Verification items for the finished model (mm, model axes). Give positions to 0.01 mm unless a question says otherwise; leave off trailing zeros. Write each loop counter-clockwise with the first axis right and the second up, starting at its lowest first coordinate (ties: lowest second). Pieces come first, ordered by that corner, then holes. Notation, with made-up numbers: (51.5, 63.5) -> (94.5, 63.5) arc R28 ccw to (94.5, 84.5) -> close; hole circle Ø7 at (71.5, 68.25). An arc over 180 degrees is marked (long way). Write item = value, one per line.
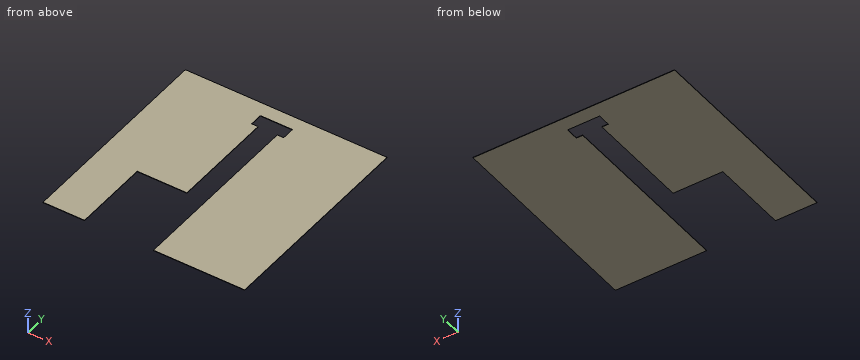
from build123d import *

# Parameters (mm, degrees)
CROQUIS1_W              = 1258.4
CROQUIS1_H              = 1300
SALIENTE_EXTRUIR1_DEPTH = 2.9
CROQUIS2_W              = 200
CROQUIS2_H              = 80
CORTAR_EXTRUIR1_DEPTH   = 10
CORTAR_EXTRUIR2_DEPTH   = 3


with BuildPart() as part:
    # Croquis1 → Saliente-Extruir1 (new body)
    with BuildSketch(Plane.XY):
        with Locations((629.2, -650)):
            Rectangle(CROQUIS1_W, CROQUIS1_H)
    extrude(amount=SALIENTE_EXTRUIR1_DEPTH)

    # Croquis2 → Cortar-Extruir1 (cut)
    with BuildSketch(Plane.XY.offset(2.9)):
        with Locations((629.2, -128.9)):
            Rectangle(CROQUIS2_W, CROQUIS2_H)
    extrude(amount=-CORTAR_EXTRUIR1_DEPTH, mode=Mode.SUBTRACT)

    # Croquis3 → Cortar-Extruir2 (cut)
    with BuildSketch(Plane.XY.offset(2.9)):
        Polygon((569.2, -168.9), (569.2, -818.9), (259.2, -818.9), (259.2, -1300), (689.2, -1300), (689.2, -168.9), align=None)
    extrude(amount=-CORTAR_EXTRUIR2_DEPTH, mode=Mode.SUBTRACT)


solid = part.part
Item 1: Go/stop test with a flat-tipped pin: P1, Ø1.5, axis at x = 581.5, z = 1.5, coming from the -Y side. Record where the tip stops, or that it passes through.
Response values:
P1 = -88.9
Item 2: Sectioned sample at A-A on y = -916. Record the cut outline in (x, z).
Response values:
outline = (0, 0) -> (259.2, 0) -> (259.2, 2.9) -> (0, 2.9) -> close; (689.2, 0) -> (1258.4, 0) -> (1258.4, 2.9) -> (689.2, 2.9) -> close
Item 3: Material ranges on line 1 (X direction, y = -176, z = 1.2); line 2 (X direction, y = -1092.5, z = 1.95); line 3 (Y direction, x = 530.5, z = 1.05), recorded low to high.
Response values:
line_1 = 0 to 569.2, 689.2 to 1258.4
line_2 = 0 to 259.2, 689.2 to 1258.4
line_3 = -818.9 to -168.9, -88.9 to 0
Item 4: Sectioned sample at D-D on x = 653. Record the cut outline in (y, z).
Response values:
outline = (-88.9, 0) -> (0, 0) -> (0, 2.9) -> (-88.9, 2.9) -> close
Item 5: Sectioned sample at C-C on y = -497. Record the cut outline in (x, z), then the cut area to 3 significant figures.
Response values:
outline = (0, 0) -> (569.2, 0) -> (569.2, 2.9) -> (0, 2.9) -> close; (689.2, 0) -> (1258.4, 0) -> (1258.4, 2.9) -> (689.2, 2.9) -> close
area = 3,300 mm^2
Item 6: Sectioned sample at B-B on z = 1.1. Record the cut outline in (x, y).
Response values:
outline = (0, -1300) -> (259.2, -1300) -> (259.2, -818.9) -> (569.2, -818.9) -> (569.2, -168.9) -> (529.2, -168.9) -> (529.2, -88.9) -> (729.2, -88.9) -> (729.2, -168.9) -> (689.2, -168.9) -> (689.2, -1300) -> (1258.4, -1300) -> (1258.4, 0) -> (0, 0) -> close
